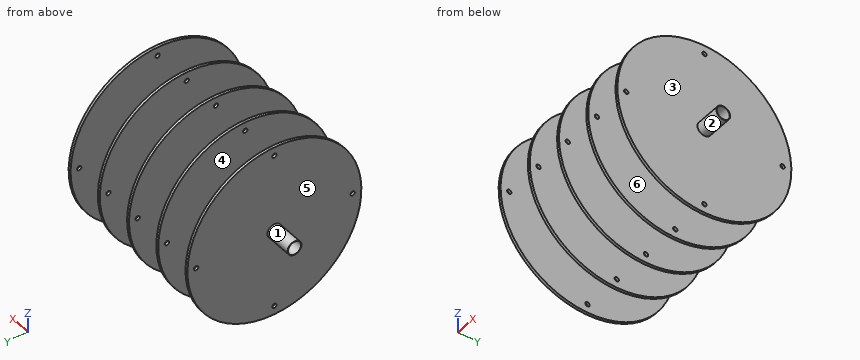
from build123d import *

# Parameters (mm, degrees)
SKETCH1_R                  = 8
SKETCH1_R_2                = 7.5
BOSS_EXTRUDE1_DEPTH        = 121.5
SKETCH2_R                  = 100
BOSS_EXTRUDE2_DEPTH        = 3
SKETCH3_R                  = 2.5
CUT_EXTRUDE1_DEPTH         = 257.507309837
CIRPATTERN1_COUNT          = 4
LPATTERN1_COUNT            = 5
LPATTERN1_PITCH            = 45
LPATTERN1_COPY_1_SKETCH_R  = 2.5
LPATTERN1_COPY_1_DEPTH     = 257.507309837
LPATTERN1_COPY_2_SKETCH_R  = 2.5
LPATTERN1_COPY_2_DEPTH     = 257.507309837
LPATTERN1_COPY_3_SKETCH_R  = 2.5
LPATTERN1_COPY_3_DEPTH     = 257.507309837
LPATTERN1_COPY_4_SKETCH_R  = 2.5
LPATTERN1_COPY_4_DEPTH     = 257.507309837
LPATTERN1_COPY_5_SKETCH_R  = 2.5
LPATTERN1_COPY_5_DEPTH     = 257.507309837
LPATTERN1_COPY_6_SKETCH_R  = 2.5
LPATTERN1_COPY_6_DEPTH     = 257.507309837
LPATTERN1_COPY_7_SKETCH_R  = 2.5
LPATTERN1_COPY_7_DEPTH     = 257.507309837
LPATTERN1_COPY_8_SKETCH_R  = 2.5
LPATTERN1_COPY_8_DEPTH     = 257.507309837
LPATTERN1_COPY_9_SKETCH_R  = 2.5
LPATTERN1_COPY_9_DEPTH     = 257.507309837
LPATTERN1_COPY_10_SKETCH_R = 2.5
LPATTERN1_COPY_10_DEPTH    = 257.507309837
LPATTERN1_COPY_11_SKETCH_R = 2.5
LPATTERN1_COPY_11_DEPTH    = 257.507309837
LPATTERN1_COPY_12_SKETCH_R = 2.5
LPATTERN1_COPY_12_DEPTH    = 257.507309837


with BuildPart() as part:
    # Sketch1 → Boss-Extrude1 (new, symmetric)
    with BuildSketch(Plane(origin=(0, 0, 0), x_dir=(0, 0, -1), z_dir=(1, 0, 0))):
        Circle(SKETCH1_R)
        Circle(SKETCH1_R_2, mode=Mode.SUBTRACT)
    extrude(amount=BOSS_EXTRUDE1_DEPTH, both=True)

    # Sketch2 → Boss-Extrude2 (add)
    with BuildSketch(Plane(origin=(92.5, 0, 0), x_dir=(0, 0, -1), z_dir=(1, 0, 0))):
        Circle(SKETCH2_R)
    boss_extrude2 = extrude(amount=-BOSS_EXTRUDE2_DEPTH)

    # Sketch3 → Cut-Extrude1 (cut, through all)
    with BuildSketch(Plane(origin=(92.5, 0, 0), x_dir=(0, 0, -1), z_dir=(1, 0, 0))):
        with Locations((0, 90)):
            Circle(SKETCH3_R)
    cut_extrude1 = extrude(amount=-CUT_EXTRUDE1_DEPTH, mode=Mode.SUBTRACT)

    # CirPattern1: Cut-Extrude1 ×4 about axis
    cirpattern1_axis = Axis((0, 0, 0), (1, 0, 0))
    for i in range(1, CIRPATTERN1_COUNT):
        add(cut_extrude1.rotate(cirpattern1_axis, i * 360 / CIRPATTERN1_COUNT), mode=Mode.SUBTRACT)

    # LPattern1: Boss-Extrude2, Cut-Extrude1 ×5
    with Locations(*[(-i * LPATTERN1_PITCH, 0, 0) for i in range(1, LPATTERN1_COUNT)]):
        add(boss_extrude2)
        add(cut_extrude1, mode=Mode.SUBTRACT)

    # LPattern1 copy 1 sketch → LPattern1 copy 1 (cut, through all)
    with BuildSketch(Plane.YZ.offset(47.5)):
        with Locations((0, 90)):
            Circle(LPATTERN1_COPY_1_SKETCH_R)
    extrude(amount=-LPATTERN1_COPY_1_DEPTH, mode=Mode.SUBTRACT)

    # LPattern1 copy 2 sketch → LPattern1 copy 2 (cut, through all)
    with BuildSketch(Plane.YZ.offset(2.5)):
        with Locations((0, 90)):
            Circle(LPATTERN1_COPY_2_SKETCH_R)
    extrude(amount=-LPATTERN1_COPY_2_DEPTH, mode=Mode.SUBTRACT)

    # LPattern1 copy 3 sketch → LPattern1 copy 3 (cut, through all)
    with BuildSketch(Plane.YZ.offset(-42.5)):
        with Locations((0, 90)):
            Circle(LPATTERN1_COPY_3_SKETCH_R)
    extrude(amount=-LPATTERN1_COPY_3_DEPTH, mode=Mode.SUBTRACT)

    # LPattern1 copy 4 sketch → LPattern1 copy 4 (cut, through all)
    with BuildSketch(Plane.YZ.offset(-87.5)):
        with Locations((0, 90)):
            Circle(LPATTERN1_COPY_4_SKETCH_R)
    extrude(amount=-LPATTERN1_COPY_4_DEPTH, mode=Mode.SUBTRACT)

    # LPattern1 copy 5 sketch → LPattern1 copy 5 (cut, through all)
    with BuildSketch(Plane(origin=(47.5, 0, 0), x_dir=(0, 0, 1), z_dir=(1, 0, 0))):
        with Locations((0, 90)):
            Circle(LPATTERN1_COPY_5_SKETCH_R)
    extrude(amount=-LPATTERN1_COPY_5_DEPTH, mode=Mode.SUBTRACT)

    # LPattern1 copy 6 sketch → LPattern1 copy 6 (cut, through all)
    with BuildSketch(Plane(origin=(2.5, 0, 0), x_dir=(0, 0, 1), z_dir=(1, 0, 0))):
        with Locations((0, 90)):
            Circle(LPATTERN1_COPY_6_SKETCH_R)
    extrude(amount=-LPATTERN1_COPY_6_DEPTH, mode=Mode.SUBTRACT)

    # LPattern1 copy 7 sketch → LPattern1 copy 7 (cut, through all)
    with BuildSketch(Plane(origin=(-42.5, 0, 0), x_dir=(0, 0, 1), z_dir=(1, 0, 0))):
        with Locations((0, 90)):
            Circle(LPATTERN1_COPY_7_SKETCH_R)
    extrude(amount=-LPATTERN1_COPY_7_DEPTH, mode=Mode.SUBTRACT)

    # LPattern1 copy 8 sketch → LPattern1 copy 8 (cut, through all)
    with BuildSketch(Plane(origin=(-87.5, 0, 0), x_dir=(0, 0, 1), z_dir=(1, 0, 0))):
        with Locations((0, 90)):
            Circle(LPATTERN1_COPY_8_SKETCH_R)
    extrude(amount=-LPATTERN1_COPY_8_DEPTH, mode=Mode.SUBTRACT)

    # LPattern1 copy 9 sketch → LPattern1 copy 9 (cut, through all)
    with BuildSketch(Plane(origin=(47.5, 0, 0), x_dir=(0, -1, 0), z_dir=(1, 0, 0))):
        with Locations((0, 90)):
            Circle(LPATTERN1_COPY_9_SKETCH_R)
    extrude(amount=-LPATTERN1_COPY_9_DEPTH, mode=Mode.SUBTRACT)

    # LPattern1 copy 10 sketch → LPattern1 copy 10 (cut, through all)
    with BuildSketch(Plane(origin=(2.5, 0, 0), x_dir=(0, -1, 0), z_dir=(1, 0, 0))):
        with Locations((0, 90)):
            Circle(LPATTERN1_COPY_10_SKETCH_R)
    extrude(amount=-LPATTERN1_COPY_10_DEPTH, mode=Mode.SUBTRACT)

    # LPattern1 copy 11 sketch → LPattern1 copy 11 (cut, through all)
    with BuildSketch(Plane(origin=(-42.5, 0, 0), x_dir=(0, -1, 0), z_dir=(1, 0, 0))):
        with Locations((0, 90)):
            Circle(LPATTERN1_COPY_11_SKETCH_R)
    extrude(amount=-LPATTERN1_COPY_11_DEPTH, mode=Mode.SUBTRACT)

    # LPattern1 copy 12 sketch → LPattern1 copy 12 (cut, through all)
    with BuildSketch(Plane(origin=(-87.5, 0, 0), x_dir=(0, -1, 0), z_dir=(1, 0, 0))):
        with Locations((0, 90)):
            Circle(LPATTERN1_COPY_12_SKETCH_R)
    extrude(amount=-LPATTERN1_COPY_12_DEPTH, mode=Mode.SUBTRACT)


solid = part.part
Could you check a few things on this model? Use its own coordinates, in mm. Face numbers are marked on the shaded views. A direction names the side the tool comes from. Give positions to 0.01 mm unless a question says otherwise; leave off trailing zeros. Loops run counter-clockwise (first coordinate to the right, second up) from the corner with the lowest first, then second, coordinate; pieces in that order, holes last. Notation, with made-up numbers: (50, 79.25) -> (68, 79.25) arc R17 cw to (68, 87.25) -> close; hole circle Ø10 at (71.5, 30.5). An arc over 180 degrees is marked (long way). Answer as CSV lines item,"result". Start each with the question number.
(1) Which directions (+Z, -Z, +X, -X, +Y, -Y) give clear straight access to the entire face, cutting with the end or side of a thin tool? Please do the marked faces 1 and 2.
(2) I need wall thicknesses on probe 1 along X at (y, z) = (-78, 47.5); probe 2 along Y at (x, z) = (-89, 0); probe 3 along Z at (x, y) = (20.5, 4). Which ranges of each line are inside material? Lowest first, please.
(3) If we section it at A-A on y = -39.5: Write out the boundary of the cut face in (x, z).
(4) If we section it at C-C on x = -7.5: Write out the boundary of the cut face in (y, z).
(5) We'd pull the mould along X, two halves only. Please class the marked faces 3, 4, 5 and 6: released by +X, released by -X, zero draft, split by the parting line, or undercut.
(6) If we section it at B-B on z = 16.5: Write out the boundary of the cut face in (x, y).
(7) I'm going to push flat-ended pins straight in: pin 1 Ø4.5 at (y, z) = (-90, 0) entering from +X; pin 2 Ø8 at (y, z) = (0, 90) entering from +X; pin 3 Ø1 at (x, z) = (46.5, 33.5) entering from +Y; pin 4 Ø8 at (y, z) = (90, 0) entering from -X. Where does each tip first touch, or does it pass through?
Computed:
1,face 1,"-X"
1,face 2,"+X"
2,probe 1,"x = -90.5 to -87.5, -45.5 to -42.5, -0.5 to 2.5, 44.5 to 47.5, 89.5 to 92.5"
2,probe 2,"y = -100 to -92.5, -87.5 to 87.5, 92.5 to 100"
2,probe 3,"z = -6.93 to -6.34, 6.34 to 6.93"
3,outline,"(-90.5, -91.87) -> (-87.5, -91.87) -> (-87.5, 91.87) -> (-90.5, 91.87) -> close; (-45.5, -91.87) -> (-42.5, -91.87) -> (-42.5, 91.87) -> (-45.5, 91.87) -> close; (-0.5, -91.87) -> (2.5, -91.87) -> (2.5, 91.87) -> (-0.5, 91.87) -> close; (44.5, -91.87) -> (47.5, -91.87) -> (47.5, 91.87) -> (44.5, 91.87) -> close; (89.5, -91.87) -> (92.5, -91.87) -> (92.5, 91.87) -> (89.5, 91.87) -> close"
4,outline,"circle Ø16 at (0, 0); hole circle Ø15 at (0, 0)"
5,face 3,"released by +X"
5,face 4,"undercut"
5,face 5,"released by -X"
5,face 6,"undercut"
6,outline,"(-90.5, -98.63) -> (-87.5, -98.63) -> (-87.5, 98.63) -> (-90.5, 98.63) -> close; (-45.5, -98.63) -> (-42.5, -98.63) -> (-42.5, 98.63) -> (-45.5, 98.63) -> close; (-0.5, -98.63) -> (2.5, -98.63) -> (2.5, 98.63) -> (-0.5, 98.63) -> close; (44.5, -98.63) -> (47.5, -98.63) -> (47.5, 98.63) -> (44.5, 98.63) -> close; (89.5, -98.63) -> (92.5, -98.63) -> (92.5, 98.63) -> (89.5, 98.63) -> close"
7,pin 1,"passes through"
7,pin 2,"stops at x = 92.5"
7,pin 3,"stops at y = 94.4"
7,pin 4,"stops at x = -90.5"
